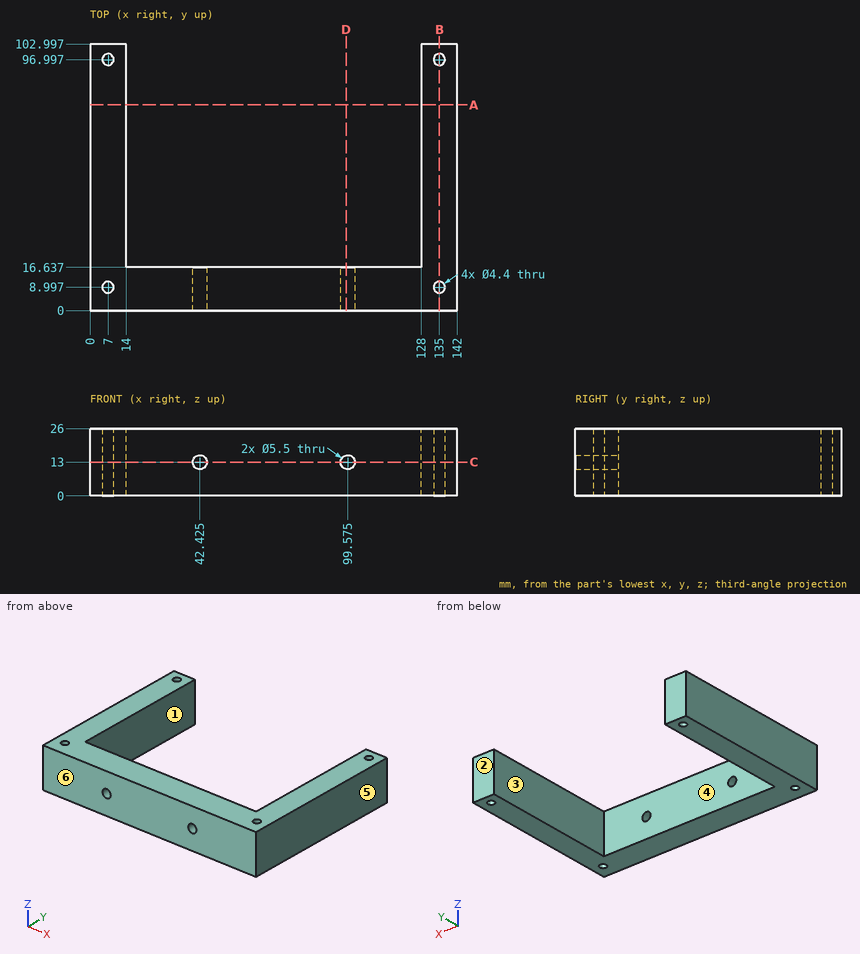
Can you work these out from the drawing? Everything is in mm from the part's minimum corner. A direction names the side the tool comes from. Give positions to 0.01 mm unless a question says otherwise; leave off trailing zeros. Write each loop counter-clockwise with the first axis right and the second up, starting at its lowest first coordinate (ties: lowest second). Pieces come first, ordered by that corner, then holes. Notation, with made-up numbers: M 48,36.5 L 57,36.5 A23 ccw 57,45.5 Z; hole C 15.5,-19 d9. An arc over 180 degrees is marked long. Answer in a Markdown table with one row per item. Add a question column.
Item 1: Imagine slicing it at D-D, the plane x = 99. Write out the boundary of the cut face in (y, z).
Item 2: Imagine slicing it at A-A, the plane y = 79.5. Write out the boundary of the cut face in (x, z).
Item 3: For pin 1 Ø5 at (x, y) = (135, 96.997) entering from +Z; pin 2 Ø7 at (x, z) = (99.575, 13) entering from +Y, each with a flat end and sliding along its axis, tell me the tip position at first contact or that it passes through.
Item 4: Imagine slicing it at B-B, the plane x = 135. Write out the boundary of the cut face in (y, z), plus the area to 3 significant figures.
Item 5: Imagine slicing it at C-C, the plane z = 13. Write out the boundary of the cut face in (x, y) (3 decimals).
Item 6: On a 3-axis mill with a long thin cutter (end or side, diameter ignored), from which of +Z, -Z, +X, -X, +Y, -Y can I reach the whole of each face in a straight line? I mean the marked faces 1 and 2. Say none if no direction works.
Item 7: We'd pull the mould along X, two halves only. Please class the marked faces 3, 4, 5 and 6: released by +X, released by -X, zero draft, split by the parting line, or undercut.
Item 8: Please list where these lines run through material, in increasing order: L1, parallel to Y at x = 7, z = 19.5; L2, parallel to X at y = 89, z = 19; L3, parallel to X at y = 8.25, z = 13 (3 decimals).
Evaluation:
| question | item | result |
|---|---|---|
| 1 | outline | M 0,0 L 16.64,0 L 16.64,10.31 L 0,10.31 Z; M 0,15.69 L 16.64,15.69 L 16.64,26 L 0,26 Z |
| 2 | outline | M 0,0 L 14,0 L 14,26 L 0,26 Z; M 128,0 L 142,0 L 142,26 L 128,26 Z |
| 3 | pin 1 | stops at z = 26 |
| 3 | pin 2 | stops at y = 16.64 |
| 4 | outline | M 0,0 L 6.8,0 L 6.8,26 L 0,26 Z; M 11.2,0 L 94.8,0 L 94.8,26 L 11.2,26 Z; M 99.2,0 L 103,0 L 103,26 L 99.2,26 Z |
| 4 | area | 2,450 mm² |
| 5 | outline | M 0,0 L 39.675,0 L 39.675,16.637 L 14,16.637 L 14,102.997 L 0,102.997 Z; M 45.175,0 L 96.825,0 L 96.825,16.637 L 45.175,16.637 Z; M 102.325,0 L 142,0 L 142,102.997 L 128,102.997 L 128,16.637 L 102.325,16.637 Z; hole C 7,8.997 d4.4; hole C 7,96.997 d4.4; hole C 135,8.997 d4.4; hole C 135,96.997 d4.4 |
| 6 | face 1 | +Z, -Z, +Y |
| 6 | face 2 | +Z, -Z, +X, -X, +Y |
| 7 | face 3 | undercut |
| 7 | face 4 | undercut |
| 7 | face 5 | released by +X |
| 7 | face 6 | zero draft |
| 8 | L1 | y = 0 to 6.8, 11.2 to 94.8, 99.2 to 103 |
| 8 | L2 | x = 0 to 14, 128 to 142 |
| 8 | L3 | x = 0 to 4.931, 9.069 to 39.675, 45.175 to 96.825, 102.325 to 132.931, 137.069 to 142 |
